from build123d import *

# Parameters (mm, degrees)
F0_R     = 4.5
F1_DEPTH = 15
F2_R     = 2.625
F3_DEPTH = 25
F2_R_2   = 3.7
F4_DEPTH = 13
F5_R     = 0.2
F6_SIZE  = 0.8


with BuildPart() as f1:
    # F0 (on Top) → F1 (new body)
    with BuildSketch(Plane.XY):
        Circle(F0_R)
    extrude(amount=F1_DEPTH)

    # F2 (on face) → F3 (cut)
    with BuildSketch(Plane.XY.offset(15)):
        Circle(F2_R)
    extrude(amount=-F3_DEPTH, mode=Mode.SUBTRACT)

    # F2 (on face) → F4 (cut)
    with BuildSketch(Plane.XY.offset(15)):
        Circle(F2_R_2)
        Circle(F2_R, mode=Mode.SUBTRACT)
    extrude(amount=-F4_DEPTH, mode=Mode.SUBTRACT)

    # F5
    f5_edges = [f1.edges().sort_by_distance(p)[0] for p in [
        (-4.5, 0, 15),
        (-3.7, 0, 15),
        (-4.5, 0, 0),
    ]]
    fillet(f5_edges, radius=F5_R)

    # F6
    f6_edges = [f1.edges().sort_by_distance(p)[0] for p in [
        (-2.625, 0, 0),
    ]]
    chamfer(f6_edges, length=F6_SIZE)


solid = f1.part
Build history of the part. All positions in model axes, mm. A direction names the side the tool comes from. Round coordinates to 2 decimals unless told otherwise and drop trailing zeros. Write each loop counter-clockwise with the first axis right and the second up, starting at its lowest first coordinate (ties: lowest second). Pieces come first, ordered by that corner, then holes. Notation, with made-up numbers: (-24, 79) - (-4, 79) arc R14 ccw to (-4, 100) - close; hole circle Ø4 at (52.5, 84). An arc over 180 degrees is marked (long way). Use CSV: the item, a comma, the result in double quotes.
(1) Wall check: line 1 (Y direction, x = 0, z = 1.35) (3 decimals); line 2 (Y direction, x = 0, z = 8.5); line 3 (X direction, y = 3.25, z = 14). Give the ranges that are in metal, low to high.
Response:
line 1,"-4.5 to -2.625, 2.625 to 4.5"
line 2,"-4.5 to -3.7, 3.7 to 4.5"
line 3,"-3.11 to -1.77, 1.77 to 3.11"
(2) Band-saw the part on C-C (z = 1.5). Write the cut outline in (x, y) (3 decimals).
Response:
outline,"circle Ø9 at (0, 0); hole circle Ø5.25 at (0, 0)"
(3) Band-saw the part on D-D (z = 6). Write the cut outline in (x, y), plus the area to 3 significant figures.
Response:
outline,"circle Ø9 at (0, 0); hole circle Ø7.4 at (0, 0)"
area,"20.6 mm²"
(4) Pin check, flat tips, straight feed: P1, Ø3, axis at y = 2.5, z = 3.5, coming from the -X side; P2, Ø5, axis at x = -0.5, y = 0, coming from the +Z side. Stop position of each tip, or through.
Response:
P1,"x = -4.39"
P2,"z = 2"
(5) 3-axis set-ups, long thin cutter, end or side, ignore diameter. For faces 1 (the flat face through (-3, -2, 0)), 2 (the flat face through (1, 3, 2)): which of +Z, -Z, +X, -X, +Y, -Y reach the whole face in a straight line?
Response:
face 1,"-Z, +X, -X, +Y, -Y"
face 2,"+Z"
(6) Mould opens along Y. For faces 3 (the cylindrical face through (-0.802, -3.612, 8.49)), 4 (the cylindrical face through (-0.59, 4.46, 7.4)), 5 (the flat face through (1, -4, 15)) say: pulls with the +Y half, pulls with the -Y half, needs draft (parallel to the pull), parting line crosses it, or undercut.
Response:
face 3,"undercut"
face 4,"parting line crosses it"
face 5,"needs draft"
(7) Band-saw the part on A-A (y = 0). Write the cut outline in (x, z) (3 decimals).
Response:
outline,"(-4.5, 0.2) arc R0.2 ccw to (-4.3, 0) - (-3.425, 0) - (-2.625, 0.8) - (-2.625, 2) - (-3.7, 2) - (-3.7, 14.8) arc R0.2 ccw to (-3.9, 15) - (-4.3, 15) arc R0.2 ccw to (-4.5, 14.8) - close; (2.625, 0.8) - (3.425, 0) - (4.3, 0) arc R0.2 ccw to (4.5, 0.2) - (4.5, 14.8) arc R0.2 ccw to (4.3, 15) - (3.9, 15) arc R0.2 ccw to (3.7, 14.8) - (3.7, 2) - (2.625, 2) - close"
